Solid Edge part; units mm, degrees
sketch "Sketch1" plane through (0, 0, 0) normal (0, -1, 0) x (1, 0, 0)
  line L0 (20, -20) -> (0, -20)
  line L1 (0, 20) -> (0, -20)
  line L2 (0, 20) -> (20, 20)
  line L3 (20, 20) -> (20, 17.608)
  arc A0 (17.7179, 15.1175) -> (20, 17.608) centre (17.5, 17.608) ccw
  line L4 (17.7179, 15.1175) -> (10.0206, 14.4441)
  arc A1 (10.0206, 14.4441) -> (5, 8.965) centre (10.5, 8.965) ccw
  line L5 (5, -8.965) -> (5, 8.965)
  arc A2 (5, -8.965) -> (10.0206, -14.4441) centre (10.5, -8.965) ccw
  line L6 (17.7179, -15.1175) -> (10.0206, -14.4441)
  arc A3 (17.7179, -15.1175) -> (20, -17.608) centre (17.5, -17.608) cw
  line L7 (20, -20) -> (20, -17.608)
extrude "Protrusion1" add sketch "Sketch1" against normal blind 19.05
Work out the finished part from the listing and answer in its coordinate system (mm). A direction names the side the tool comes from. Give positions to 0.01 mm unless a question says otherwise; leave off trailing zeros. Loops run counter-clockwise (first coordinate to the right, second up) from the corner with the lowest first, then second, coordinate; pieces in that order, holes last. Notation, with made-up numbers: (32, 10) - (62, 10) arc R14 cw to (62, 25) - close; hole circle Ø10 at (20.5, -37). An arc over 180 degrees is marked (long way). Answer in a Markdown table with one row per item. Add a question column.
Q1. The part is cut by section C-C (x = 9). Determine the outline of the cut face in (y, z).
Q2. The part is cut by section D-D (z = -4.5). Determine the outline of the cut face in (x, y).
Q3. Consider line 1 along X through (y, z) = (3.5, -4); line 2 along X through (y, z) = (2.5, 17.5); line 3 along Z through (x, y) = (18.25, 1.25). Determine where each line is inside the solid, lowest interval first.
Q4. The part is cut by section A-A (x = 14.5). Determine the outline of the cut face in (y, z).
Q5. The part is cut by section B-B (y = 3.25). Determine the outline of the cut face in (x, z) (3 decimals).
Q6. A tool of negligible diameter and unlimited length cuts with its end or side. For faces 4 (the flat face through (10, 9, -20)), 5 (the cylindrical face through (6.48, 9.39, 12.72)), from which of +Z, -Z, +X, -X, +Y, -Y can it reach the whole face along a straight path? Write none if from no direction.
Q7. Each of these flat-tipped pins is pushed along its axis until it touches: P1, Ø4, axis at y = 16, z = 7, coming from the +X side; P2, Ø10, axis at y = 3.5, z = 8.5, coming from the +X side; P3, Ø1.5, axis at y = 12.5, z = 11.5, coming from the +X side. Where does it stop, or does it pass through?
Q8. Determine the mould class of faces 1 (the flat face through (10, 9, 20)), 2 (the flat face through (13.923, 9.392, 14.786)), 3 (the flat face through (3, 0, 0)) for opening direction Z: released by +Z, released by -Z, zero draft, split by the parting line, or undercut.
Solution:
| question | item | result |
|---|---|---|
| 1 | outline | (0, -20) - (19.05, -20) - (19.05, -14.26) - (0, -14.26) - close; (0, 14.26) - (19.05, 14.26) - (19.05, 20) - (0, 20) - close |
| 2 | outline | (0, 0) - (5, 0) - (5, 19.05) - (0, 19.05) - close |
| 3 | line 1 | x = 0 to 5 |
| 3 | line 2 | x = 0 to 20 |
| 3 | line 3 | z = -20 to -15.22, 15.22 to 20 |
| 4 | outline | (0, -20) - (19.05, -20) - (19.05, -14.84) - (0, -14.84) - close; (0, 14.84) - (19.05, 14.84) - (19.05, 20) - (0, 20) - close |
| 5 | outline | (0, -20) - (20, -20) - (20, -17.608) arc R2.5 ccw to (17.718, -15.118) - (10.021, -14.444) arc R5.5 cw to (5, -8.965) - (5, 8.965) arc R5.5 cw to (10.021, 14.444) - (17.718, 15.118) arc R2.5 ccw to (20, 17.608) - (20, 20) - (0, 20) - close |
| 6 | face 4 | -Z, +X, -X, +Y, -Y |
| 6 | face 5 | +X, +Y, -Y |
| 7 | P1 | stops at x = 5 |
| 7 | P2 | stops at x = 7.39 |
| 7 | P3 | stops at x = 6.09 |
| 8 | face 1 | released by +Z |
| 8 | face 2 | undercut |
| 8 | face 3 | zero draft |
